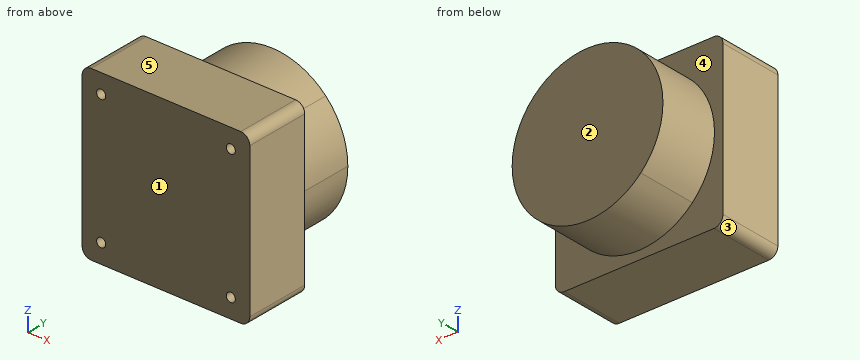
from build123d import *

# Parameters (mm, degrees)
SKETCH_1_W          = 55.6
SKETCH_1_H          = 55.6
EXTRUDE_1_DEPTH     = 21.3
EXTRUDE_2_DEPTH     = 20
FILLET_1_R          = 3
HOLE_WIZARD_1_D     = 3
HOLE_WIZARD_1_DEPTH = 4


with BuildPart() as part:
    # 草图1 → 凸台-拉伸1 (new body)
    with BuildSketch(Plane(origin=(0, 0, 0), x_dir=(1, 0, 0), z_dir=(0, 1, 0))):
        with Locations((27.8, 27.8)):
            Rectangle(SKETCH_1_W, SKETCH_1_H)
    extrude(amount=EXTRUDE_1_DEPTH)

    # 草图2 → 凸台-拉伸2 (add)
    with BuildSketch(Plane(origin=(0, 21.3, 0), x_dir=(1, 0, 0), z_dir=(0, 1, 0))):
        with BuildLine():
            ThreePointArc((52.8, 27.8), (37.367085809, 50.896988313), (10.12233047, 45.47766953))
            Line((10.12233047, 45.47766953), (45.47766953, 10.12233047))
            ThreePointArc((45.47766953, 10.12233047), (50.896988313, 18.232914191), (52.8, 27.8))
        make_face()
        with BuildLine():
            Line((45.47766953, 10.12233047), (10.12233047, 45.47766953))
            ThreePointArc((10.12233047, 45.47766953), (10.12233047, 10.12233047), (45.47766953, 10.12233047))
        make_face()
    extrude(amount=EXTRUDE_2_DEPTH)

    # 圆角1
    fillet_1_edges = [part.edges().sort_by_distance(p)[0] for p in [
        (0, 10.65, -55.6),
        (55.6, 10.65, -55.6),
        (55.6, 10.65, 0),
        (0, 10.65, 0),
    ]]
    fillet(fillet_1_edges, radius=FILLET_1_R)

    # 孔1
    with Locations(Plane(origin=(0, 0, 0), x_dir=(-1, 0, 0), z_dir=(0, -1, 0))):
        with Locations((-49.3, 49.3), (-6.3, 49.3), (-6.3, 6.3), (-49.3, 6.3)):
            Hole(HOLE_WIZARD_1_D / 2, depth=HOLE_WIZARD_1_DEPTH)


solid = part.part
Check sheet for the modelled part. Datum: model origin and axes. Units: mm. Face numbers are marked on the shaded views. A direction names the side the tool comes from. Give positions to 0.01 mm unless a question says otherwise; leave off trailing zeros. Loops run counter-clockwise (first coordinate to the right, second up) from the corner with the lowest first, then second, coordinate; pieces in that order, holes last. Notation, with made-up numbers: M 54.5,1.25 L 91.5,1.25 A33 ccw 91.5,38.25 Z; hole C 4.5,71 d1. An arc over 180 degrees is marked long. Return JSON: item names as keys, results as strings. Group by question number.
1. Tool access check on the marked faces 4 and 5. Record the directions out of +Z, -Z, +X, -X, +Y, -Y that give a thin tool (end or side, any length) a straight path to the whole face; none if there is none.
2. Go/stop test with flat-tipped pins: pin 1 (0.9 mm diameter, centred on x = 50, z = -7, fed in from -Y); pin 2 (2.5 mm diameter, centred on x = 49.3, z = -6.3, fed in from +Y); pin 3 (12 mm diameter, centred on x = 12, y = 31.5, fed in from +Z). Record where each tip stops, or that it passes through.
3. Cross-section at B-B on x = 27.8. Record the boundary of the cut face in (y, z).
4. Cross-section at D-D on x = 6.3. Record the boundary of the cut face in (y, z).
5. Cross-section at A-A on z = -19. Record the boundary of the cut face in (x, y).
6. Thickness scan on L1, parallel to Z at x = 49.3, y = 1.9; L2, parallel to X at y = 1, z = -6; L3, parallel to Y at x = 45.5, z = -48.5. Record the ranges inside material, lowest first.
7. Cross-section at C-C on y = 35. Record the boundary of the cut face in (x, z), plus the area to 3 significant figures.
8. Mould release check, pull along Y, two halves, no side actions. Record for the marked faces 1, 2 and 3: released by +Y, released by -Y, zero draft, split by the parting line, or undercut.
Return value:
{
 "1": {"face 4": "+Y", "face 5": "+Z, +X, -X, +Y, -Y"},
 "2": {"pin 1": "y = 4", "pin 2": "y = 21.3", "pin 3": "z = -4.8"},
 "3": {"outline": "M 0,-55.6 L 21.3,-55.6 L 21.3,-52.8 L 41.3,-52.8 L 41.3,-2.8 L 21.3,-2.8 L 21.3,0 L 0,0 Z"},
 "4": {"outline": "M 0,-55.6 L 21.3,-55.6 L 21.3,-40.56 L 41.3,-40.56 L 41.3,-15.04 L 21.3,-15.04 L 21.3,0 L 0,0 L 0,-4.8 L 4,-4.8 L 4,-7.8 L 0,-7.8 L 0,-47.8 L 4,-47.8 L 4,-50.8 L 0,-50.8 Z"},
 "5": {"outline": "M 0,0 L 55.6,0 L 55.6,21.3 L 51.2,21.3 L 51.2,41.3 L 4.4,41.3 L 4.4,21.3 L 0,21.3 Z"},
 "6": {"L1": "-55.6 to -50.8, -47.8 to -7.8, -4.8 to 0", "L2": "0 to 4.83, 7.77 to 47.83, 50.77 to 55.6", "L3": "0 to 21.3"},
 "7": {"outline": "C 27.8,-27.8 d50", "area": "1,960 mm^2"},
 "8": {"face 1": "released by -Y", "face 2": "released by +Y", "face 3": "zero draft"}
}
